Verification items for the finished model (mm, model axes). Face numbers are marked on the shaded views. A direction names the side the tool comes from. Coordinates: 2 decimals unless noted, no trailing zeros. Write each loop counter-clockwise with the first axis right and the second up, starting at its lowest first coordinate (ties: lowest second). Pieces come first, ordered by that corner, then holes. Notation, with made-up numbers: (44, -16) - (84, -16) arc R22 ccw to (84, -6) - close; hole circle Ø7 at (3, 63.25). An arc over 180 degrees is marked (long way). Use one line per item in the form item = value. Start each with the question number.
(1) Sectioned sample at D-D (x = 5). Record the cut outline in (y, z), and give its area (3 significant figures).
(2) Tool access check on the marked faces 1, 2 and 3. Record the directions out of +Z, -Z, +X, -X, +Y, -Y that give a thin tool (end or side, any length) a straight path to the whole face; none if there is none.
(3) Sectioned sample at A-A (y = 0). Record the cut outline in (x, z), and give its area (3 significant figures).
(4) Material ranges on line 1 (Z direction, x = 25, y = -0.25); line 2 (Y direction, x = 9, z = -2.75), recorded low to high. Write a range as [from, to].
(5) Gauge pin test, flat ends, axial feed: pin 1 Ø4 at (x, z) = (19, 5) entering from +Y; pin 2 Ø2 at (x, y) = (15.5, 0) entering from +Z; pin 3 Ø3 at (y, z) = (-5.5, -4.5) entering from -X. Record the tip position at first contact, or that the pin passes through.
(6) Sectioned sample at C-C (x = 36.5). Record the cut outline in (y, z), and give its area (3 significant figures).
from build123d import *

# Parameters (mm, degrees)
SKETCH2_W           = 8.128
SKETCH2_H           = 8.128
BOSS_EXTRUDE1_DEPTH = 4.7625


with BuildPart() as part:
    # Sketch1 → Revolve1 (revolve)
    with BuildSketch(Plane.XY, mode=Mode.PRIVATE) as revolve1_sk:
        with BuildLine():
            Line((3.9704, 9.1313), (4.4704, 9.1313))
            Line((4.4704, 9.1313), (4.4704, 3.81))
            Line((4.4704, 3.81), (9.2329, 3.81))
            Line((9.2329, 3.81), (9.2329, 3.96875))
            Line((9.2329, 3.96875), (55.2704, 3.96875))
            Line((55.2704, 3.96875), (55.2704, 0))
            Line((55.2704, 0), (0, 0))
            ThreePointArc((0, 0), (1.035543925, 4.97857198), (3.9704, 9.1313))
        make_face()
    revolve(revolve1_sk.sketch.rotate(Axis((0, 0, 0), (-1, 0, 0)), 90), axis=Axis((0, 0, 0), (-1, 0, 0)))

    # Sketch2 → Boss-Extrude1 (add)
    with BuildSketch(Plane(origin=(4.4704, 0, 0), x_dir=(0, 0, -1), z_dir=(1, 0, 0))):
        Rectangle(SKETCH2_W, SKETCH2_H)
    extrude(amount=BOSS_EXTRUDE1_DEPTH)


solid = part.part
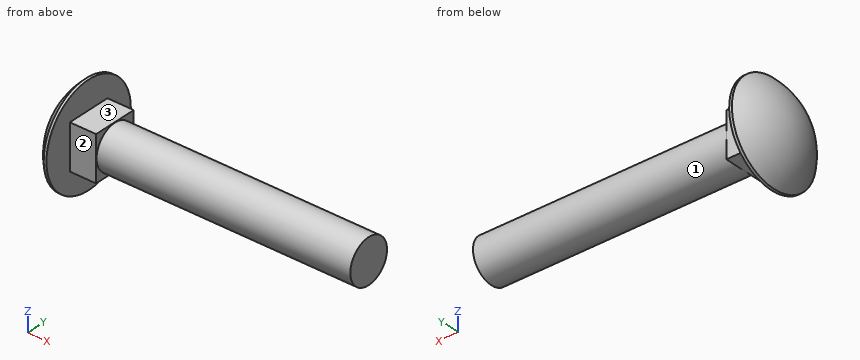
Answers below:
q1.outline = (-4.06, -4.06) - (4.06, -4.06) - (4.06, 4.06) - (-4.06, 4.06) - close
q1.area = 66.1 mm2
q2.face_1 = +X
q2.face_2 = +Z, -Z, +X, -Y
q2.face_3 = +Z, +X, +Y, -Y
q3.outline = (3.97, -9.13) - (4.47, -9.13) - (4.47, -4.06) - (9.23, -4.06) - (9.23, -3.97) - (55.27, -3.97) - (55.27, 3.97) - (9.23, 3.97) - (9.23, 4.06) - (4.47, 4.06) - (4.47, 9.13) - (3.97, 9.13) arc R12.49 ccw to start
q3.area = 463 mm2
q4.line_1 = [-3.96, 3.96]
q4.line_2 = [-4.06, 4.06]
q5.pin_1 = 2.6
q5.pin_2 = 3.97
q5.pin_3 = 1.33
q6.outline = circle Ø7.94 at (0, 0)
q6.area = 49.5 mm2
